Design review of the part built by this model. Coordinates are the model's own, in mm. A direction names the side the tool comes from. Round coordinates to 2 decimals unless told otherwise and drop trailing zeros. Write each loop counter-clockwise with the first axis right and the second up, starting at its lowest first coordinate (ties: lowest second). Pieces come first, ordered by that corner, then holes.
from build123d import *

# Parameters (mm, degrees)
EXTRUDE_THIN2_DEPTH     = 165.4
SKETCH11_W              = 166
SKETCH11_H              = 4
BOSS_EXTRUDE3_DEPTH     = 2.6416
CUT_EXTRUDE6_DEPTH      = 270.69086006
CUT_EXTRUDE6_DEPTH_BACK = 270.69086006
SKETCH13_W              = 110.495011338
SKETCH13_H              = 5
CUT_EXTRUDE7_DEPTH      = 273.127102656
SKETCH19_W              = 4
SKETCH19_H              = 155.4
CUT_EXTRUDE9_DEPTH      = 10
SKETCH20_W              = 4
SKETCH20_H              = 155.4
CUT_EXTRUDE10_DEPTH     = 10
SKETCH21_W              = 6
SKETCH21_H              = 86.697
BOSS_EXTRUDE4_DEPTH     = 110
CUT_EXTRUDE11_DEPTH     = 4
SKETCH23_W              = 166
SKETCH23_H              = 4
BOSS_EXTRUDE5_DEPTH     = 2.6416


with BuildPart() as part:
    # Sketch2 → Extrude-Thin2 (new body)
    with BuildSketch(Plane.XY):
        Polygon((0, 120), (0, 0), (186, 0), (186, 120), (176, 120), (176, 10), (10, 10), (10, 120), align=None)
    extrude(amount=EXTRUDE_THIN2_DEPTH)

    # Sketch11 → Boss-Extrude3 (add)
    with BuildSketch(Plane(origin=(0, 10, 0), x_dir=(1, 0, 0), z_dir=(0, 1, 0))):
        with Locations((93, -34.703)):
            Rectangle(SKETCH11_W, SKETCH11_H)
    extrude(amount=BOSS_EXTRUDE3_DEPTH)

    # Sketch13 → Cut-Extrude6 (cut, two sides: drawn at the far end of the back side and taken through both)
    with BuildSketch(Plane(origin=(10, 0, 0), x_dir=(0, 0, -1), z_dir=(1, 0, 0)).offset(-CUT_EXTRUDE6_DEPTH_BACK)):
        with Locations((-103.947505669, 89.551599899)):
            Rectangle(SKETCH13_W, SKETCH13_H)
    extrude(amount=CUT_EXTRUDE6_DEPTH + CUT_EXTRUDE6_DEPTH_BACK, mode=Mode.SUBTRACT)

    # Sketch14 → Cut-Extrude7 (cut, through all)
    with BuildSketch(Plane(origin=(0, 10, 0), x_dir=(1, 0, 0), z_dir=(0, 1, 0))):
        with BuildLine():
            Line((176, -165.4), (10, -165.4))
            ThreePointArc((10, -165.4), (93, -135.4), (176, -165.4))
        make_face()
    extrude(amount=-CUT_EXTRUDE7_DEPTH, mode=Mode.SUBTRACT)

    # Sketch19 → Cut-Extrude9 (cut)
    with BuildSketch(Plane(origin=(0, 120, 0), x_dir=(1, 0, 0), z_dir=(0, 1, 0))):
        with Locations((5, -82.7)):
            Rectangle(SKETCH19_W, SKETCH19_H)
    extrude(amount=-CUT_EXTRUDE9_DEPTH, mode=Mode.SUBTRACT)

    # Sketch20 → Cut-Extrude10 (cut)
    with BuildSketch(Plane(origin=(0, 120, 0), x_dir=(1, 0, 0), z_dir=(0, 1, 0))):
        with Locations((181, -82.7)):
            Rectangle(SKETCH20_W, SKETCH20_H)
    extrude(amount=-CUT_EXTRUDE10_DEPTH, mode=Mode.SUBTRACT)

    # Sketch21 → Boss-Extrude4 (add, through all)
    with BuildSketch(Plane(origin=(0, 10, 0), x_dir=(1, 0, 0), z_dir=(0, 1, 0))):
        with Locations((93, -82.0515)):
            Rectangle(SKETCH21_W, SKETCH21_H)
    extrude(amount=BOSS_EXTRUDE4_DEPTH)

    # Sketch22 → Cut-Extrude11 (cut)
    with BuildSketch(Plane(origin=(0, 10, 0), x_dir=(1, 0, 0), z_dir=(0, 1, 0))):
        Polygon((36, -48.703), (36, -148.583194008), (42, -145.837577441), (42, -48.703), align=None)
        Polygon((144, -145.837577441), (150, -148.583194008), (150, -48.703), (144, -48.703), align=None)
    extrude(amount=-CUT_EXTRUDE11_DEPTH, mode=Mode.SUBTRACT)

    # Sketch23 → Boss-Extrude5 (add)
    with BuildSketch(Plane(origin=(0, 10, 0), x_dir=(1, 0, 0), z_dir=(0, 1, 0))):
        with Locations((93, -27.4)):
            Rectangle(SKETCH23_W, SKETCH23_H)
    extrude(amount=BOSS_EXTRUDE5_DEPTH)


solid = part.part
1) Add section C-C on z = 86.5. Count the separate pieces of the cut face and the enclosed holes in it, and give its area (3 significant figures).
2) For faces 4 (the face through (181, 90, 159.195)), 5 (the face through (93, 64, 125.4)), 6 (the face through (3, 115, 84)), list the 3-axis set-ups (+Z, -Z, +X, -X, +Y, -Y) from which the entire face can be reached by the end or side of a thin tool; tool diameter is ignored.
3) For line 1 along X through (y, z) = (35, 115.5); line 2 along X through (y, z) = (113, 72.5); line 3 along X through (y, z) = (40, 158.5), list the stretches that pass through material, from the lowest coordinate up.
4) For P1, Ø4, axis at x = 122.5, z = 46, coming from the +Y side; P2, Ø6.5, axis at x = 94, y = 80, coming from the +Z side; P3, Ø12, axis at x = 28, z = 33.5, coming from the +Y side, all flat-tipped, find the tip position at first contact; note any pin that passes through.
5) Add section B-B on z = 45. State the section outline as (x, y) points, and give its area (3 significant figures).
6) Add section D-D on x = 110.5. State the section outline as (y, z) points.
7) Add section A-A on y = 53. State the section outline as (x, z) points.
8) The part is to be moulded in two halves that separate along Y. For faces 1 (the face through (181, 92.052, 105)), 2 (the face through (176, 66, 82)), 3 (the face through (147, 6, 98)), say which applies: pulls with the +Y half, pulls with the -Y half, needs draft (parallel to the pull), parting line crosses it, or undercut.
Computed:
1. separate pieces: 3
1. enclosed holes: 0
1. area: 4,490 mm2
2. face 4: +X, -X
2. face 5: +Z, +Y
2. face 6: +Y
3. line 1: x = 0 to 10, 90 to 96, 176 to 186
3. line 2: x = 0 to 3, 7 to 10, 90 to 96, 176 to 179, 183 to 186
3. line 3: x = 0 to 10, 176 to 186
4. P1: stops at y = 10
4. P2: stops at z = 125.4
4. P3: stops at y = 12.64
5. outline: (0, 0) - (186, 0) - (186, 120) - (183, 120) - (183, 110) - (179, 110) - (179, 120) - (176, 120) - (176, 10) - (96, 10) - (96, 120) - (90, 120) - (90, 10) - (10, 10) - (10, 120) - (7, 120) - (7, 110) - (3, 110) - (3, 120) - (0, 120) - close
5. area: 4,640 mm2
6. outline: (0, 0) - (10, 0) - (10, 25.4) - (12.64, 25.4) - (12.64, 29.4) - (10, 29.4) - (10, 32.7) - (12.64, 32.7) - (12.64, 36.7) - (10, 36.7) - (10, 136.58) - (0, 136.58) - close
7. outline: (0, 0) - (10, 0) - (10, 165.4) - (0, 165.4) - close; (90, 38.7) - (96, 38.7) - (96, 125.4) - (90, 125.4) - close; (176, 0) - (186, 0) - (186, 165.4) - (176, 165.4) - close
8. face 1: undercut
8. face 2: needs draft
8. face 3: pulls with the +Y half
